Geometry check sheet. Reference: the model listing, model coordinates, mm. Round coordinates to 2 decimals unless told otherwise and drop trailing zeros. Loops run counter-clockwise (first coordinate to the right, second up) from the corner with the lowest first, then second, coordinate; pieces in that order, holes last. Notation, with made-up numbers: (9, 35.5) -> (46, 35.5) arc R15 ccw to (46, 51.5) -> close; hole circle Ø3 at (-36.75, 52.25). An arc over 180 degrees is marked (long way). Use a Markdown table: item, result. Add a question column.
Q1. Material ranges on L1, parallel to Y at x = -120.65, z = -1.7 (3 decimals); L2, parallel to X at y = 166.5, z = -1.5; L3, parallel to Y at x = -77.5, z = -0.6 (3 decimals), recorded low to high.
Q2. Sectioned sample at C-C, the plane z = -1.65. Give the number of separate pieces and of enclosed holes in the cut face, then the cut area to 3 significant figures.
Q3. Sectioned sample at A-A, the plane x = -25.4. Enter the section's corners in (y, z) (3 decimals).
Q4. Release check for a two-part mould opening along X. For faces 1 (the face through (-121.141, 125.963, -1.565)), 2 (the face through (-74, 92, -3.175)), 3 (the face through (-76.561, 78.256, -1.565)) record: released by +X, released by -X, zero draft, split by the parting line, or undercut.
Q5. Sectioned sample at B-B, the plane x = -120.65. Enter the section's corners in (y, z) (3 decimals).
Q6. Gauge pin test, flat end, axial feed: P1, Ø20.5, axis at x = -33.782, y = 19.685, coming from the +Z side. Record the tip position at first contact, or that the pin passes through.
```python
from build123d import *

# Parameters (mm, degrees)
SKETCH1_W                        = 146.05
SKETCH1_H                        = 180.975
BOSS_EXTRUDE1_DEPTH              = 3.175
F_6_CLEARANCE_HOLE1_D            = 4.3053
F_19_64_0_29688_DIAMETER_HOLE1_D = 7.540752
F_1_2_0_5_DIAMETER_HOLE1_D       = 12.7
F_5_32_0_15625_DIAMETER_HOLE1_D  = 3.96875
F_3_32_0_09375_DIAMETER_HOLE1_D  = 2.38125


with BuildPart() as part:
    # Sketch1 → Boss-Extrude1 (new body)
    with BuildSketch(Plane.XY):
        with Locations((-73.025, 90.4875)):
            Rectangle(SKETCH1_W, SKETCH1_H)
    extrude(amount=-BOSS_EXTRUDE1_DEPTH)

    # #6 Clearance Hole1 (through all)
    with Locations(Plane(origin=(0, 0, -3.175), x_dir=(-1, 0, 0), z_dir=(0, 0, -1))):
        with Locations((25.4, 142.875), (73.025, 142.875), (127, 142.875), (25.4, 34.925), (73.025, 61.647038728), (127, 34.925), (4.8895, 14.2875), (141.1605, 14.2875), (4.8895, 90.4875), (141.1605, 90.4875), (141.1605, 166.6875), (4.8895, 166.6875)):
            Hole(F_6_CLEARANCE_HOLE1_D / 2)

    # 19/64 (0.29688) Diameter Hole1 (through all)
    with Locations(Plane(origin=(0, 0, -3.175), x_dir=(-1, 0, 0), z_dir=(0, 0, -1))):
        with Locations((25.4, 160.3248), (57.15, 160.3248), (88.9, 160.3248), (120.65, 160.3248), (25.4, 122.2248), (57.15, 122.2248), (88.9, 122.2248), (120.65, 122.2248)):
            Hole(F_19_64_0_29688_DIAMETER_HOLE1_D / 2)

    # 1/2 (0.5) Diameter Hole1 (through all)
    with Locations(Plane(origin=(0, 0, -3.175), x_dir=(-1, 0, 0), z_dir=(0, 0, -1))):
        with Locations((75.184, 84.455), (119.888, 84.455), (119.888, 52.07), (33.782, 52.07), (33.782, 19.685), (119.888, 19.685), (76.454, 31.496)):
            Hole(F_1_2_0_5_DIAMETER_HOLE1_D / 2)

    # 5/32 (0.15625) Diameter Hole1 (through all)
    with Locations(Plane(origin=(0, 0, -3.175), x_dir=(-1, 0, 0), z_dir=(0, 0, -1))):
        with Locations((72.963204011, 18.468172011)):
            Hole(F_5_32_0_15625_DIAMETER_HOLE1_D / 2)

    # 3/32 (0.09375) Diameter Hole1 (through all)
    with Locations(Plane(origin=(0, 0, -3.175), x_dir=(-1, 0, 0), z_dir=(0, 0, -1))):
        with Locations((19.4, 160.324800026), (51.15, 160.324800026), (82.9, 160.324800026), (114.65, 160.324800026), (114.65, 122.224800026), (82.9, 122.224800026), (51.15, 122.224800026), (19.4, 122.224800026)):
            Hole(F_3_32_0_09375_DIAMETER_HOLE1_D / 2)


solid = part.part
```
Values:
| question | item | result |
|---|---|---|
| 1 | L1 | 0 to 13.381, 25.989 to 45.766, 58.374 to 78.151, 90.759 to 118.454, 125.995 to 156.554, 164.095 to 180.975 |
| 1 | L2 | -146.05 to -143.3, -139.02 to -7.03, -2.75 to 0 |
| 1 | L3 | 0 to 25.233, 37.759 to 78.542, 90.368 to 180.975 |
| 2 | separate pieces | 1 |
| 2 | enclosed holes | 36 |
| 2 | area | 25,000 mm^2 |
| 3 | outline | (0, -3.175) -> (32.772, -3.175) -> (32.772, 0) -> (0, 0) -> close; (37.078, -3.175) -> (118.454, -3.175) -> (118.454, 0) -> (37.078, 0) -> close; (125.995, -3.175) -> (140.722, -3.175) -> (140.722, 0) -> (125.995, 0) -> close; (145.028, -3.175) -> (156.554, -3.175) -> (156.554, 0) -> (145.028, 0) -> close; (164.095, -3.175) -> (180.975, -3.175) -> (180.975, 0) -> (164.095, 0) -> close |
| 4 | face 1 | undercut |
| 4 | face 2 | zero draft |
| 4 | face 3 | undercut |
| 5 | outline | (0, -3.175) -> (13.381, -3.175) -> (13.381, 0) -> (0, 0) -> close; (25.989, -3.175) -> (45.766, -3.175) -> (45.766, 0) -> (25.989, 0) -> close; (58.374, -3.175) -> (78.151, -3.175) -> (78.151, 0) -> (58.374, 0) -> close; (90.759, -3.175) -> (118.454, -3.175) -> (118.454, 0) -> (90.759, 0) -> close; (125.995, -3.175) -> (156.554, -3.175) -> (156.554, 0) -> (125.995, 0) -> close; (164.095, -3.175) -> (180.975, -3.175) -> (180.975, 0) -> (164.095, 0) -> close |
| 6 | P1 | z = 0 |
